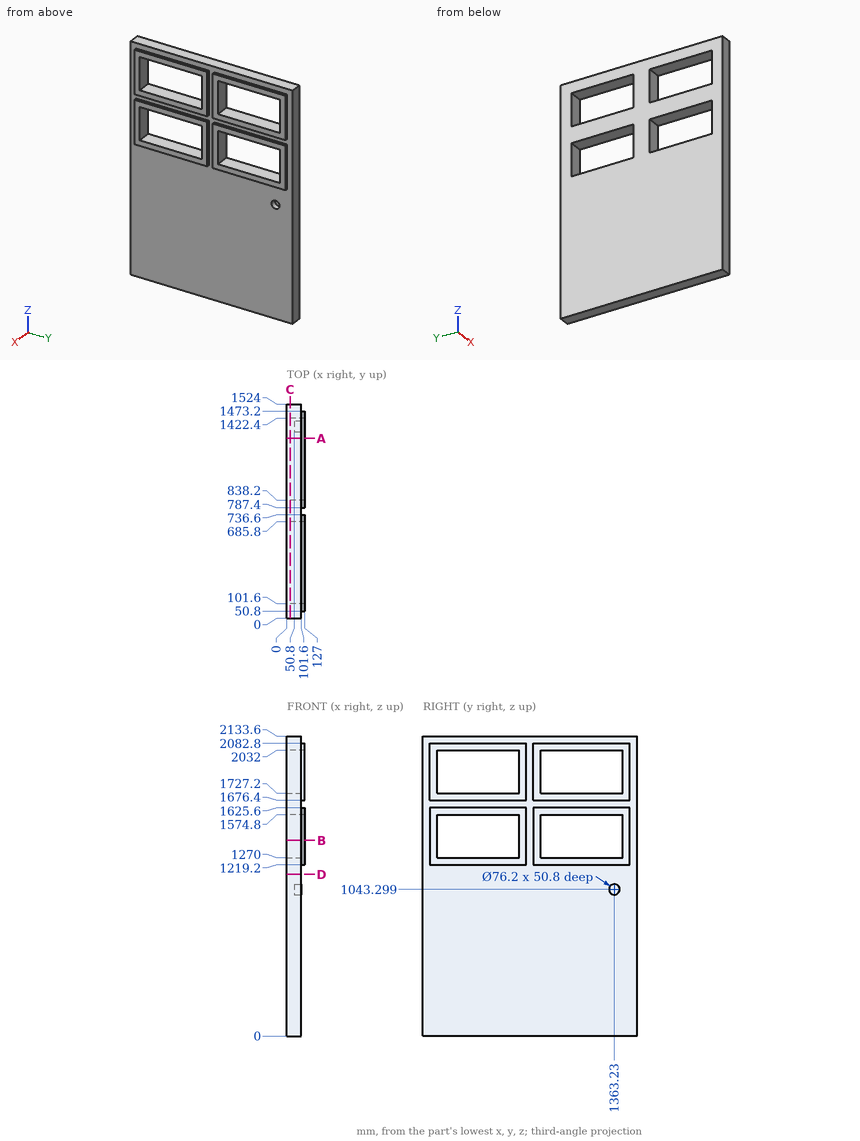
Print and shaded views of the part. All mm, measured from the part's lowest x, y and z. Give positions to 0.01 mm unless a question says otherwise; leave off trailing zeros. Write each loop counter-clockwise with the first axis right and the second up, starting at its lowest first coordinate (ties: lowest second). Pieces come first, ordered by that corner, then holes. Notation, with made-up numbers: (40, -12) -> (55, -12) arc R17 ccw to (55, 5) -> close; hole circle Ø11 at (39.25, -18). An arc over 180 degrees is marked (long way). Use CSV: the item, a comma, the result in double quotes. Start each with the question number.
1) Drill centre lines: L1, parallel to Z at x = 113, y = 252; L2, parallel to Z at x = 99.5, y = 667.5; L3, parallel to Y at x = 53.5, z = 1529. Where is each one in solid material? Low to high.
2) Cut at A-A on y = 1278.5. List the corners of the cut face in (x, z).
3) Cut at D-D on z = 1149.5. List the corners of the cut face in (x, y).
4) Cut at B-B on z = 1391.5. List the corners of the cut face in (x, y).
5) Pin check, flat tips, straight feed: P1, Ø20.5, axis at x = 118.5, y = 1038, coming from the -Z side; P2, Ø4, axis at y = 338, z = 389, coming from the +X side; P3, Ø20.5, axis at x = 116.5, z = 1789.5, coming from the +Y side. Stop position of each tip, or through.
6) Cut at C-C on x = 22. List the corners of the cut face in (y, z).
Final values:
1,L1,"z = 1219.2 to 1270, 1574.8 to 1625.6, 1676.4 to 1727.2, 2032 to 2082.8"
1,L2,"z = 0 to 1270, 1574.8 to 1727.2, 2032 to 2133.6"
1,L3,"y = 0 to 101.6, 685.8 to 838.2, 1422.4 to 1524"
2,outline,"(0, 0) -> (101.6, 0) -> (101.6, 1219.2) -> (127, 1219.2) -> (127, 1270) -> (0, 1270) -> close; (0, 1574.8) -> (127, 1574.8) -> (127, 1625.6) -> (101.6, 1625.6) -> (101.6, 1676.4) -> (127, 1676.4) -> (127, 1727.2) -> (0, 1727.2) -> close; (0, 2032) -> (127, 2032) -> (127, 2082.8) -> (101.6, 2082.8) -> (101.6, 2133.6) -> (0, 2133.6) -> close"
3,outline,"(0, 0) -> (101.6, 0) -> (101.6, 1524) -> (0, 1524) -> close"
4,outline,"(0, 0) -> (101.6, 0) -> (101.6, 50.8) -> (127, 50.8) -> (127, 101.6) -> (0, 101.6) -> close; (0, 685.8) -> (127, 685.8) -> (127, 736.6) -> (101.6, 736.6) -> (101.6, 787.4) -> (127, 787.4) -> (127, 838.2) -> (0, 838.2) -> close; (0, 1422.4) -> (127, 1422.4) -> (127, 1473.2) -> (101.6, 1473.2) -> (101.6, 1524) -> (0, 1524) -> close"
5,P1,"stops at z = 1219.2"
5,P2,"stops at x = 101.6"
5,P3,"stops at y = 1473.2"
6,outline,"(0, 0) -> (1524, 0) -> (1524, 2133.6) -> (0, 2133.6) -> close; hole (101.6, 1270) -> (685.8, 1270) -> (685.8, 1574.8) -> (101.6, 1574.8) -> close; hole (101.6, 1727.2) -> (685.8, 1727.2) -> (685.8, 2032) -> (101.6, 2032) -> close; hole (838.2, 1270) -> (1422.4, 1270) -> (1422.4, 1574.8) -> (838.2, 1574.8) -> close; hole (838.2, 1727.2) -> (1422.4, 1727.2) -> (1422.4, 2032) -> (838.2, 2032) -> close"
